Work out the finished part from the listing and answer in its coordinate system (mm). Coordinates: 2 decimals unless noted, no trailing zeros. Write each loop counter-clockwise with the first axis right and the second up, starting at its lowest first coordinate (ties: lowest second). Pieces come first, ordered by that corner, then holes. Notation, with made-up numbers: (70, 18) - (122, 18) arc R18 cw to (122, 26) - close; hole circle Ø4 at (52, 54.5). An arc over 180 degrees is marked (long way). One line per item, written item: value.
Autodesk Inventor part; units mm, degrees
ref_plane "YZ Plane" through (0, 0, 0) normal (1, 0, 0) x (0, 1, 0)
ref_plane "XZ Plane" through (0, 0, 0) normal (0, 1, 0) x (-1, 0, 0)
ref_plane "XY Plane" through (0, 0, 0) normal (0, 0, 1) x (1, 0, 0)
sketch "Sketch1" plane through (0, 0, 0) normal (0, 0, 1) x (1, 0, 0)
  line L0 (-661.6722, 0) -> (196.8414, 0)
  line L1 (0, -264.4179) -> (0, 989.622)
  line L2 (0, 0) -> (-137.5064, 137.5064) construction
  circle A0 centre (0, 0) radius 17.78
  line L3 (0, 0) -> (46.0238, 46.0238) construction
  line L4 (-64.8398, 5.6727) -> (0, 0) construction
  circle A1 centre (-64.8398, 5.6727) radius 6.35 construction
  circle A2 centre (46.0238, 46.0238) radius 6.35 construction
  arc A3 (52.7316, 41.7801) -> (45.7909, 53.9579) centre (46.0238, 46.0238) ccw
  arc A4 (-69.7613, 11.9003) -> (-67.2505, -1.8898) centre (-64.8398, 5.6727) ccw
  line L5 (0, 0) -> (3.2586, 111.9917) construction
  line L6 (0, 0) -> (-89.6909, 100.7848) construction
  arc A5 (-69.7613, 11.9003) -> (-35.8824, 40.3207) centre (-539.0274, 605.7002) ccw
  arc A6 (1.5698, 53.9522) -> (45.7909, 53.9579) centre (23.5824, 810.4734) ccw
  arc A7 (-50.976, -17.7412) -> (-67.2505, -1.8898) centre (-74.9647, -26.0901) ccw
  arc A8 (52.7316, 41.7801) -> (50.4537, 19.1761) centre (74.1966, 28.2002) ccw
  arc A9 (1.5698, 53.9522) -> (-35.8824, 40.3207) centre (0, 0) ccw
  line L7 (-43.1182, -37.2395) -> (-51.5426, -60.3852)
  line L8 (9.0934, -56.243) -> (0.6691, -79.3887)
  arc A10 (-48.7265, -68.0701) -> (-6.4279, -83.4655) centre (17.2205, 47.3129) ccw
  arc A11 (-50.976, -17.7412) -> (-43.9184, -31.3763) centre (0, 0) ccw
  arc A12 (13.4752, -52.2659) -> (50.4537, 19.1761) centre (0, 0) ccw
  line L9 (-28.2338, -77.5716) -> (0, 0) construction
  arc A13 (-43.1182, -37.2395) -> (-43.9184, -31.3763) centre (-49.0853, -35.0676) ccw
  arc A14 (13.4752, -52.2659) -> (9.0934, -56.243) centre (15.0605, -58.4148) ccw
  arc A15 (-6.4279, -83.4655) -> (0.6691, -79.3887) centre (-5.298, -77.2168) ccw
  arc A16 (-51.5426, -60.3852) -> (-48.7265, -68.0701) centre (-45.5755, -62.557) ccw
  circle A17 centre (-17.0625, 17.0625) radius 4.7625
  circle A18 centre (0, 0) radius 16.51 construction
  point P0 (-41.9333, -33.9838)
  point P1 (-53.3354, -65.3108)
  point P2 (-1.1237, -84.3143)
  point P3 (10.2784, -52.9873)
  dimension "d1" = 45
  dimension "d2" = 35.56
  dimension "d33" = 45
  dimension "d34" = 65.0875
  dimension "d39" = 65.0875
  dimension "d40" = 12.7
  dimension "d41" = 130
  dimension "d42" = 1.5875
  dimension "d43" = 1.5875
  dimension "d44" = 43.333
  dimension "d46" = 86.667
  dimension "d47" = 25.4
  dimension "d48" = 53.975
  dimension "d70" = 53.975
  dimension "d71" = 53.975
  dimension "d72" = 20
  dimension "d74" = 33.3375
  dimension "d75" = 33.3375
  dimension "d76" = 82.55
  dimension "d77" = 27.7812
  dimension "d78" = 6.35
  dimension "d89" = 24.13
  dimension "d90" = 9.525
  dimension "d91" = 33.02
extrude "Base" add sketch "Sketch1" along normal mid plane 6.35 contours A4 A5 A9 L1 A0 L0 | L0 A0 L1 A15 A10 A16 L7 A13 A11 A7 A4 | L1 A9 A6 A3 A8 A12 L0 A0 | A0 L0 A12 A14 L8 A15 L1
sketch "Sketch3" plane through (0, 0, 3.175) normal (0, 0, 1) x (1, 0, 0)
  line L0 (0, 0) -> (-18.7854, 40.2854) construction
  line L1 (-98.1278, 0) -> (79.3255, 0)
  line L2 (0, -111.0752) -> (0, 81.4834)
  point P0 (-40.2854, -18.7854)
  point P1 (18.7854, -40.2854)
  point P2 (40.2854, 18.7854)
  dimension "d20" = 44.45
  dimension "d23" = 360
  dimension "d57" = 25
hole "Motor Mount Holes" at (-18.7854, 40.2854, 3.175) at (-40.2854, -18.7854, 3.175) at (18.7854, -40.2854, 3.175) at (40.2854, 18.7854, 3.175) direction (0, 0, -1) diameter 5.1054 end through all countersink diameter 9.779 countersink angle 82
sketch "Sketch4" plane through (0, 0, -3.175) normal (0, 0, -1) x (-1, 0, 0)
  arc A0 (67.2505, -1.8898) -> (69.7613, 11.9003) centre (64.8398, 5.6727) ccw
  arc A1 (-45.7909, 53.9579) -> (-52.7316, 41.7801) centre (-46.0238, 46.0238) ccw
hole "Standoff holes to back plate" at (46.0238, 46.0238, -3.175) at (-64.8398, 5.6727, -3.175) direction (0, 0, 1) diameter 5.1054 end through all counterbore diameter 9.779 counterbore depth 1.5875
sketch "Sketch5" plane through (0, 0, 3.175) normal (0, 0, 1) x (1, 0, 0)
  circle A0 centre (-64.8398, 5.6727) radius 2.5527
  circle A1 centre (46.0238, 46.0238) radius 2.5527
  circle A2 centre (-52.2014, -3.9338) radius 6.35 construction
  circle A3 centre (42.5172, 30.5409) radius 6.35 construction
  arc A4 (1.5698, 53.9522) -> (-35.8824, 40.3207) centre (0, 0) ccw
  line L0 (-52.2014, -3.9338) -> (0, 0) construction
  line L1 (-98.1278, 0) -> (79.3255, 0)
  line L2 (0, -111.7873) -> (0, 85.7561)
  line L3 (0, 0) -> (42.5172, 30.5409) construction
  dimension "d58" = 15.875
  dimension "d59" = 15.875
  dimension "d60" = 12.7
  dimension "d62" = 12.7
  dimension "d92" = 52.3494
  dimension "d93" = 52.3494
hole "Standoff holes to front plate" at (-52.2014, -3.9338, 3.175) at (42.5172, 30.5409, 3.175) direction (0, 0, -1) diameter 3.683 end through all counterbore diameter 9.779 counterbore depth 1.5875
sketch "Sketch6" plane through (0, 0, 3.175) normal (0, 0, 1) x (1, 0, 0)
  arc A0 (-48.7265, -68.0701) -> (-6.4279, -83.4655) centre (17.2205, 47.3129) ccw
  line L0 (9.0934, -56.243) -> (0.6691, -79.3887)
  arc A1 (-46.8486, -63.1399) -> (-40.4997, -65.4507) centre (-43.6742, -64.2953) ccw
  arc A2 (-11.0463, -76.1709) -> (-4.6974, -78.4817) centre (-7.8719, -77.3263) ccw
  arc A3 (0.7322, -63.5641) -> (-5.6168, -61.2532) centre (-2.4423, -62.4087) ccw
  line L1 (-46.8486, -63.1399) -> (-41.4191, -48.2223)
  line L2 (-35.0701, -50.5331) -> (-40.4997, -65.4507)
  line L3 (-11.0463, -76.1709) -> (-5.6168, -61.2532)
  line L4 (0.7322, -63.5641) -> (-4.6974, -78.4817)
  line L5 (-43.6742, -64.2953) -> (-7.8719, -77.3263) construction
  arc A4 (-35.0701, -50.5331) -> (-41.4191, -48.2223) centre (-38.2446, -49.3777) ccw
  arc A5 (1.5698, 53.9522) -> (-35.8824, 40.3207) centre (0, 0) ccw
  circle A6 centre (0, 0) radius 53.975 construction
  dimension "d80" = 15.875
  dimension "d81" = 6.7564
  dimension "d82" = 5.353
  dimension "d83" = 38.1
  dimension "d84" = 2.3813
  dimension "d86" = 15.875
  dimension "d94" = 107.95
extrude "Tensioning Slots" cut sketch "Sketch6" against normal through all
equation "\"d43\" = d42"
equation "\"d44\" = 0.333333 * d41"
equation "\"d46\" = 0.666667 * d41"
properties part number "motor plate"
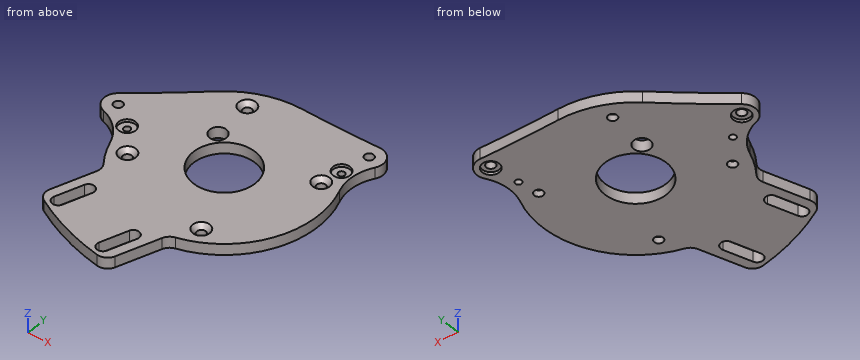
Item 1: Section A-A, the plane x = -9 is taken. Determine the outline of the cut face in (y, z) (1 decimal).
Evaluation:
outline: (-83, -3.2) - (-80.5, -3.2) - (-80.5, 3.2) - (-83, 3.2) - close; (-70.5, -3.2) - (-15.3, -3.2) - (-15.3, 3.2) - (-70.5, 3.2) - close; (15.3, -3.2) - (53.2, -3.2) - (53.2, 3.2) - (15.3, 3.2) - close
Item 2: Section C-C, the plane x = -30.5 is taken. Determine the outline of the cut face in (y, z) (1 decimal), then the cut area to 3 significant figures.
Evaluation:
outline: (-76.7, -3.2) - (44.5, -3.2) - (44.5, 3.2) - (-76.7, 3.2) - close
area: 770 mm2
Item 3: Given pin 1 (6 mm diameter, centred on x = 18.79, y = -40.29, fed in from +Z); pin 2 (1.5 mm diameter, centred on y = -66.5, z = 0.5, fed in from +X); pin 3 (3 mm diameter, centred on x = 43.5, y = 45, fed in from -Z), each flat-ended and moving along its own axis, determine where each tip first touches the part or whether it passes through.
Evaluation:
pin 1: stops at z = 1.01
pin 2: stops at x = 5.63
pin 3: stops at z = -1.59
Item 4: Consider probe 1 along X at (y, z) = (13, -2); probe 2 along X at (y, z) = (7, -2.5); probe 3 along Y at (x, z) = (-15, -1.5). Determine where each line is inside the solid, lowest interval first.
Evaluation:
probe 1: x = -68.37 to -19.55, -14.58 to -12.13, 12.13 to 52.39
probe 2: x = -72.67 to -69.55, -60.13 to -16.34, 16.34 to 53.52
probe 3: y = -81.62 to -9.55, 9.55 to 12.77, 21.36 to 51.85
Item 5: Section B-B, the plane z = -0.5 is taken. Give the number of separate pieces and of enclosed holes in the cut face, then the cut area to 3 significant figures.
Evaluation:
separate pieces: 1
enclosed holes: 12
area: 10,300 mm2
